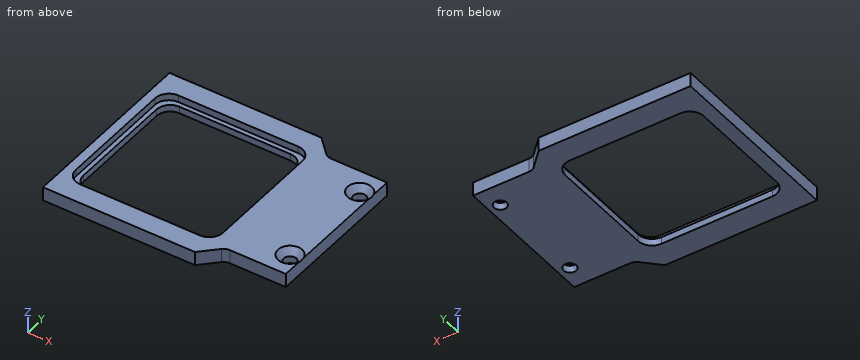
from build123d import *

# Parameters (mm, degrees)
F1_DEPTH       = 9.525
F3_DEPTH       = 4.7752
F4_DEPTH       = 9.526
F6_D           = 8.73125
F6_CSINK_D     = 16.6624
F6_CSINK_ANGLE = 82


# Not quite as in the source:
# - a length typed as a fraction of an inch, garbled in the dataset ("3 / 203.2 mm" for 3/8 in), is restored


with BuildPart() as f1:
    # F0 (on Top) → F1 (new body)
    with BuildSketch(Plane.XY):
        with BuildLine():
            Line((37.8966893194, 57.4490684102), (-66.8783106806, 57.4490684102))
            Line((-66.8783106806, 57.4490684102), (-66.8783106806, -69.5509315898))
            Line((-66.8783106806, -69.5509315898), (37.8966893194, -69.5509315898))
            Line((37.8966893194, -69.5509315898), (48.7368173799, -58.7108035293))
            ThreePointArc((48.7368173799, -58.7108035293), (50.796905645, -57.3342965584), (53.2269454405, -56.8509315898))
            Line((53.2269454405, -56.8509315898), (91.8716893194, -56.8509315898))
            Line((91.8716893194, -56.8509315898), (91.8716893194, 44.7490684102))
            Line((91.8716893194, 44.7490684102), (53.2269454405, 44.7490684102))
            ThreePointArc((53.2269454405, 44.7490684102), (50.796905645, 45.2324333787), (48.7368173799, 46.6089403496))
            Line((48.7368173799, 46.6089403496), (37.8966893194, 57.4490684102))
        make_face()
    extrude(amount=F1_DEPTH)

    # F2 (on face) → F3 (cut)
    with BuildSketch(Plane.XY.offset(9.525)):
        with BuildLine():
            Line((31.5466893194, 43.2885684102), (-51.0033106806, 43.2885684102))
            ThreePointArc((-51.0033106806, 43.2885684102), (-57.7385027714, 40.498760501), (-60.5283106806, 33.7635684102))
            Line((-60.5283106806, 33.7635684102), (-60.5283106806, -45.8654315898))
            ThreePointArc((-60.5283106806, -45.8654315898), (-57.7385027714, -52.6006236806), (-51.0033106806, -55.3904315898))
            Line((-51.0033106806, -55.3904315898), (31.5466893194, -55.3904315898))
            ThreePointArc((31.5466893194, -55.3904315898), (38.2818814102, -52.6006236806), (41.0716893194, -45.8654315898))
            Line((41.0716893194, -45.8654315898), (41.0716893194, 33.7635684102))
            ThreePointArc((41.0716893194, 33.7635684102), (38.2818814102, 40.498760501), (31.5466893194, 43.2885684102))
        make_face()
        with BuildLine():
            ThreePointArc((-57.4803106806, 30.5885684102), (-54.6905027714, 37.323760501), (-47.9553106806, 40.1135684102))
            Line((-47.9553106806, 40.1135684102), (28.4986893194, 40.1135684102))
            ThreePointArc((28.4986893194, 40.1135684102), (35.2338814102, 37.323760501), (38.0236893194, 30.5885684102))
            Line((38.0236893194, 30.5885684102), (38.0236893194, -42.6904315898))
            ThreePointArc((38.0236893194, -42.6904315898), (35.2338814102, -49.4256236806), (28.4986893194, -52.2154315898))
            Line((28.4986893194, -52.2154315898), (-47.9553106806, -52.2154315898))
            ThreePointArc((-47.9553106806, -52.2154315898), (-54.6905027714, -49.4256236806), (-57.4803106806, -42.6904315898))
            Line((-57.4803106806, -42.6904315898), (-57.4803106806, 30.5885684102))
        make_face(mode=Mode.SUBTRACT)
    extrude(amount=-F3_DEPTH, mode=Mode.SUBTRACT)

    # F4 (cut, through all): a face of the model
    f4_faces = [f1.faces().sort_by_distance(p)[0] for p in [
        (-9.7283106806, -6.0509315898, 9.525),
    ]]
    extrude(f4_faces, amount=-F4_DEPTH, mode=Mode.SUBTRACT)

    # F6 (through all)
    with Locations(Plane.XY.offset(9.525)):
        with Locations((83.9214893194, 28.8740684102), (83.9214893194, -40.9759315898)):
            CounterSinkHole(F6_D / 2, F6_CSINK_D / 2, counter_sink_angle=F6_CSINK_ANGLE)


solid = f1.part
Geometry: final body of the model. Coordinates: model frame, mm. Round coordinates to 2 decimals unless told otherwise and drop trailing zeros. Loops run counter-clockwise (first coordinate to the right, second up) from the corner with the lowest first, then second, coordinate; pieces in that order, holes last. Notation, with made-up numbers: (-11.75, -37) -> (-4.75, -37) arc R25 cw to (-4.75, 1) -> close; hole circle Ø4 at (59, 28). An arc over 180 degrees is marked (long way). One line per question, with ' | ' between items. Start each with the question number.
1. Section A-A on x = -15.5. Output: boundary loops of the cut face in (y, z) (3 decimals), and give its area (3 significant figures).
2. Contact query for flat-ended pins moving along their axis: pin 1 (5 mm diameter, centred on x = 41.5, y = -10.5, fed in from -Z); pin 2 (3 mm diameter, centred on x = 64, z = 3.5, fed in from -Y). Output: stop coordinate, or through.
3. Line query: line 1 along X through (y, z) = (-39.5, 5.25); line 2 along Y through (x, z) = (85.5, 5.25); line 3 along X through (y, z) = (-21.5, 8.75). Output: solid intervals per line, ascending. Write a range as [from, to].
4. Section D-D on x = 56.5. Output: boundary loops of the cut face in (y, z) (3 decimals), and give its area (3 significant figures).
5. Section B-B on y = 12.5. Output: boundary loops of the cut face in (x, z) (3 decimals).
6. Section C-C on z = 2.5. Output: boundary loops of the cut face in (x, y) (3 decimals).
Returned:
1) outline: (-69.551, 0) -> (-52.215, 0) -> (-52.215, 4.75) -> (-55.39, 4.75) -> (-55.39, 9.525) -> (-69.551, 9.525) -> close; (40.114, 0) -> (57.449, 0) -> (57.449, 9.525) -> (43.289, 9.525) -> (43.289, 4.75) -> (40.114, 4.75) -> close | area: 300 mm2
2) pin 1: stops at z = 0 | pin 2: stops at y = -56.85
3) line 1: x = [-66.88, -60.53], [41.07, 79.55], [88.29, 91.87] | line 2: y = [-56.85, -45.31], [-36.64, 24.54], [33.21, 44.75] | line 3: x = [-66.88, -60.53], [41.07, 91.87]
4) outline: (-56.851, 0) -> (44.749, 0) -> (44.749, 9.525) -> (-56.851, 9.525) -> close | area: 968 mm2
5) outline: (-66.878, 0) -> (-57.48, 0) -> (-57.48, 4.75) -> (-60.528, 4.75) -> (-60.528, 9.525) -> (-66.878, 9.525) -> close; (38.024, 0) -> (91.872, 0) -> (91.872, 9.525) -> (41.072, 9.525) -> (41.072, 4.75) -> (38.024, 4.75) -> close
6) outline: (-66.878, -69.551) -> (37.897, -69.551) -> (48.737, -58.711) arc R6.35 cw to (53.227, -56.851) -> (91.872, -56.851) -> (91.872, 44.749) -> (53.227, 44.749) arc R6.35 cw to (48.737, 46.609) -> (37.897, 57.449) -> (-66.878, 57.449) -> close; hole (-57.48, -42.69) arc R9.525 ccw to (-47.955, -52.215) -> (28.499, -52.215) arc R9.525 ccw to (38.024, -42.69) -> (38.024, 30.589) arc R9.525 ccw to (28.499, 40.114) -> (-47.955, 40.114) arc R9.525 ccw to (-57.48, 30.589) -> close; hole circle Ø8.731 at (83.921, -40.976); hole circle Ø8.731 at (83.921, 28.874)
